Part print with two shaded views. Sizes in mm from the minimum x, y, z corner. A direction names the side the tool comes from. Round coordinates to 2 decimals unless told otherwise and drop trailing zeros. Order: outer loops, then holes, each group sorted by start corner. A loop starts at its lowest first (then second) coordinate and runs counter-clockwise, first axis right, second up. Notation, with made-up numbers: M -25.5,65.5 L -10.5,65.5 A22 cw -10.5,80.5 Z; hole C 88,61.25 d6. An arc over 180 degrees is marked long. Return JSON: item names as keys, results as strings. Group by question number.
Item 1: Slice it at A-A on x = 14. Write the cut outline in (y, z), then the cut area to 3 significant figures.
Item 2: Pull direction Z, two halves, no side cores. Call the marked faces 4, 5 and 6: pulls with the +Z half, pulls with the -Z half, needs draft (parallel to the pull), parting line crosses it, or undercut.
Item 3: Slice it at C-C on x = 4.75. Write the cut outline in (y, z).
Item 4: Which spindle directions (+Z, -Z, +X, -X, +Y, -Y) get a long thin tool onto all of the face, cutting with end or side? Do the marked faces 1, 2 and 3. Say none if no direction does.
Item 5: Pin check, flat tips, straight feed: pin 1 Ø1 at (y, z) = (4, 8.5) entering from -X; pin 2 Ø1.5 at (x, y) = (3.5, 4.5) entering from -Z; pin 3 Ø2 at (y, z) = (2, 9.5) entering from -X; pin 4 Ø1 at (x, y) = (9.5, 8) entering from +Z. Stop position of each tip, or through.
Item 6: Slice it at D-D on z = 5.75. Write the cut outline in (x, y).
Item 7: Slice it at B-B on y = 1.25. Write the cut outline in (x, z), then the cut area to 4 significant figures.
Item 8: Probe line 1 along X through (y, z) = (0.8, 6.25); line 2 along Y through (x, z) = (11.6, 6.25); line 3 along X through (y, z) = (6.75, 3.5). List the from-to ranges inside material, lowest first.
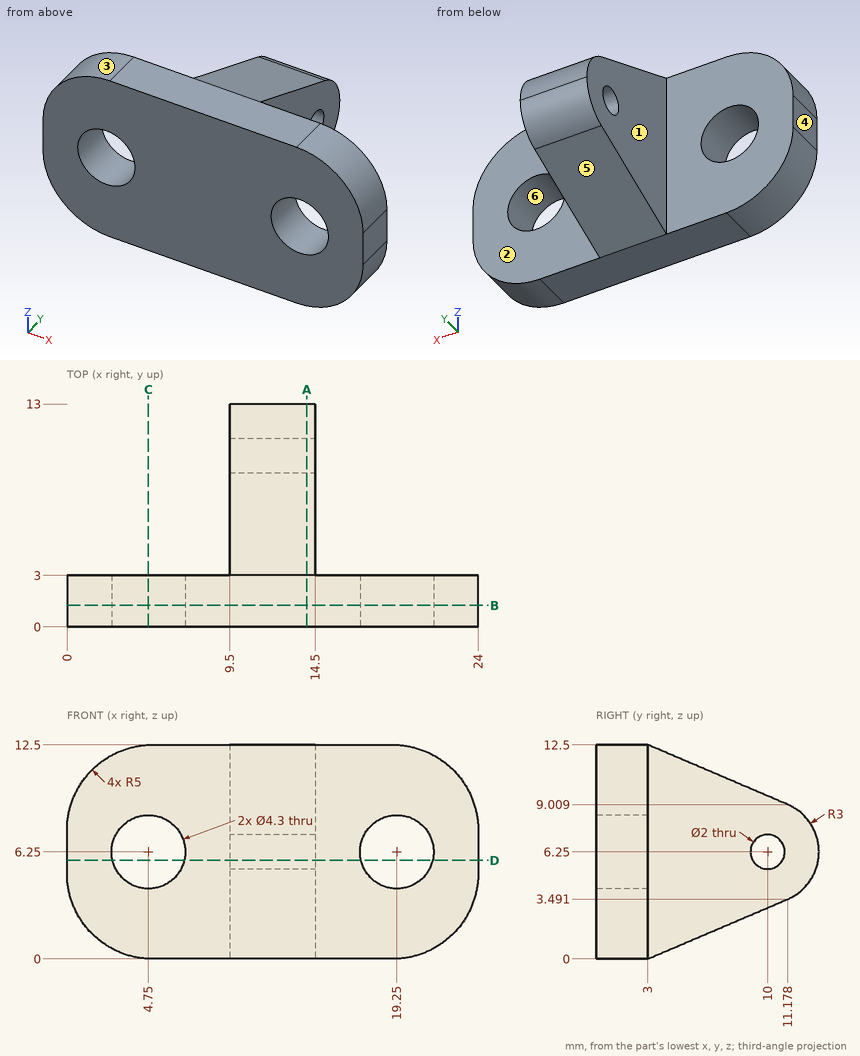
Output values:
{
 "1": {"outline": "M 0,0 L 3,0 L 11.18,3.49 A3 ccw 11.18,9.01 L 3,12.5 L 0,12.5 Z; hole C 10,6.25 d2", "area": "115 mm²"},
 "2": {"face 4": "needs draft", "face 5": "pulls with the -Z half", "face 6": "undercut"},
 "3": {"outline": "M 0,0.01 L 3,0.01 L 3,4.1 L 0,4.1 Z; M 0,8.4 L 3,8.4 L 3,12.49 L 0,12.49 Z"},
 "4": {"face 1": "+Z, -Z, -X, +Y", "face 2": "+Z, -Z, +X, +Y", "face 3": "+Z, -X, +Y, -Y"},
 "5": {"pin 1": "x = 9.5", "pin 2": "through", "pin 3": "x = 0.1", "pin 4": "z = 10.58"},
 "6": {"outline": "M 0,0 L 2.66,0 L 2.66,3 L 0,3 Z; M 6.84,0 L 17.16,0 L 17.16,3 L 14.5,3 L 14.5,9.13 L 9.5,9.13 L 9.5,3 L 6.84,3 Z; M 9.5,10.87 L 14.5,10.87 L 14.5,12.96 L 9.5,12.96 Z; M 21.34,0 L 24,0 L 24,3 L 21.34,3 Z"},
 "7": {"outline": "M 0,5 A5 ccw 5,0 L 19,0 A5 ccw 24,5 L 24,7.5 A5 ccw 19,12.5 L 5,12.5 A5 ccw 0,7.5 Z; hole C 4.75,6.25 d4.3; hole C 19.25,6.25 d4.3", "area": "249.5 mm²"},
 "8": {"line 1": "0 to 2.6, 6.9 to 17.1, 21.4 to 24", "line 2": "0 to 9, 11 to 13", "line 3": "9.5 to 14.5"}
}
